The drawing under review shows one solid part. Ordinate dimensions are in mm from its lowest x, y, z. A direction names the side the tool comes from. Round coordinates to 2 decimals unless told otherwise and drop trailing zeros. Write each loop counter-clockwise with the first axis right and the second up, starting at its lowest first coordinate (ties: lowest second). Pieces come first, ordered by that corner, then holes. Notation, with made-up numbers: M 63.25,46 L 67.25,46 A32 cw 67.25,78 Z; hole C 41,44 d6. An arc over 180 degrees is marked long. Write item = value, one per line. Start each with the question number.
Item 1: Tool access review of the marked faces 1 and 2: name each direction out of +Z, -Z, +X, -X, +Y, -Y from which nothing blocks a thin tool from reaching the whole face with its end or side.
Item 2: For pin 1 Ø3 at (x, y) = (5, 11) entering from +Z; pin 2 Ø1.7 at (y, z) = (7, 2.5) entering from +X; pin 3 Ø3 at (y, z) = (11, 4.5) entering from -X; pin 4 Ø3 at (x, y) = (1, 4.5) entering from -Z, all flat-tipped, find the tip position at first contact; note any pin that passes through.
Item 3: Take a section at B-B, the plane y = 16.5. Give the boundary of the cut face in (x, z) (3 decimals), plus the area to 3 significant figures.
Item 4: Take a section at A-A, the plane y = 4. Give the boundary of the cut face in (x, z) (3 decimals).
Item 5: To check wall thickness, follow line 1 along Z through (x, y) = (3.25, 6); line 2 along X through (y, z) = (19.25, 1.5); line 3 along X through (y, z) = (4.75, 4.75). State the ranges of each line that lie inside material, in increasing order.
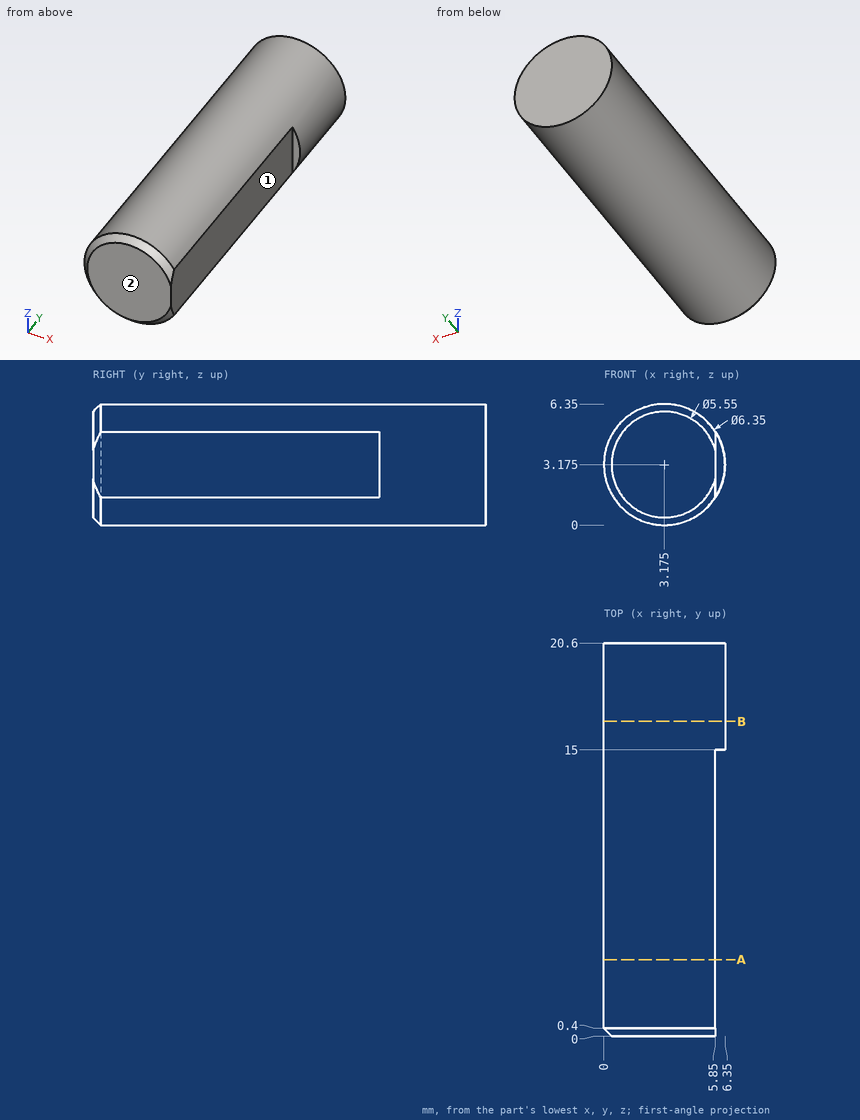
Response values:
q1.face_1 = +Z, -Z, +X, -Y
q1.face_2 = +Z, -Z, +X, -X, -Y
q2.pin_1 = 6.33
q2.pin_2 = 5.85
q2.pin_3 = 0
q2.pin_4 = 0.07
q3.outline = C 3.175,3.175 d6.35
q3.area = 31.7 mm2
q4.outline = M 5.85,1.465 L 5.85,4.885 A3.175 ccw long Z
q5.line_1 = 0 to 6.35
q5.line_2 = 0.48 to 5.87
q5.line_3 = 0.42 to 5.85
